Geometry check sheet. Reference: drawing and pictorial views, mm from the part's lowest x, y, z. A direction names the side the tool comes from. Give positions to 0.01 mm unless a question says otherwise; leave off trailing zeros. Write each loop counter-clockwise with the first axis right and the second up, starting at its lowest first coordinate (ties: lowest second). Pieces come first, ordered by that corner, then holes. Notation, with made-up numbers: (9, 77.25) -> (14, 77.25) arc R32 cw to (14, 105.25) -> close; hole circle Ø5 at (82, -38). An arc over 180 degrees is marked (long way). Return JSON: item names as keys, results as strings.
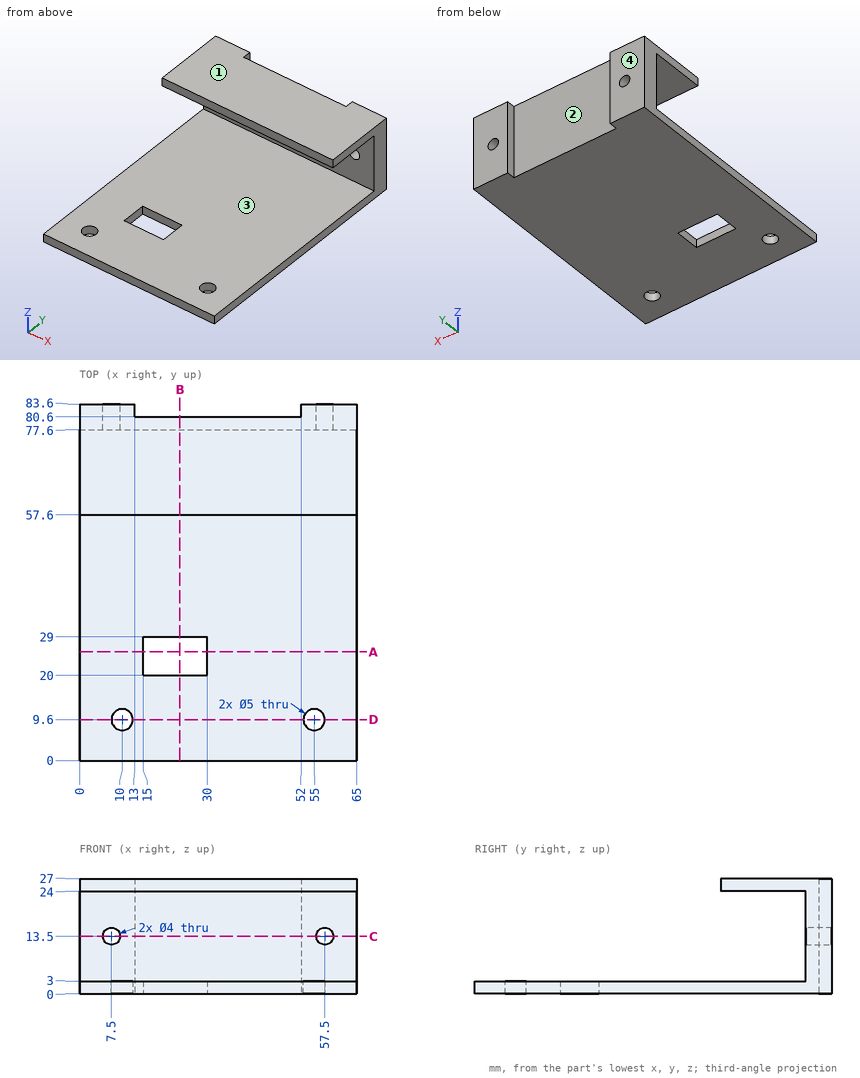
(1) Cross-section at C-C on z = 13.5. Enter the section's corners in (x, y).
Reply:
{"outline": "(0, 77.6) -> (5.5, 77.6) -> (5.5, 83.6) -> (0, 83.6) -> close; (9.5, 77.6) -> (55.5, 77.6) -> (55.5, 83.6) -> (52, 83.6) -> (52, 80.6) -> (13, 80.6) -> (13, 83.6) -> (9.5, 83.6) -> close; (59.5, 77.6) -> (65, 77.6) -> (65, 83.6) -> (59.5, 83.6) -> close"}
(2) Set-up check for the marked faces 3 and 4: record each of +Z, -Z, +X, -X, +Y, -Y from which the full face is reachable in a straight line by a thin tool's end or side.
Reply:
{"face 3": "+X, -X, -Y", "face 4": "+Z, -Z, +X, -X, +Y"}
(3) Release check for a two-part mould opening along X. For the marked faces 1 and 2 record: pulls with the +X half, pulls with the -X half, needs draft (parallel to the pull), parting line crosses it, or undercut.
Reply:
{"face 1": "needs draft", "face 2": "undercut"}
(4) Cross-section at D-D on y = 9.6. Enter the section's corners in (x, z).
Reply:
{"outline": "(0, 0) -> (7.5, 0) -> (7.5, 3) -> (0, 3) -> close; (12.5, 0) -> (52.5, 0) -> (52.5, 3) -> (12.5, 3) -> close; (57.5, 0) -> (65, 0) -> (65, 3) -> (57.5, 3) -> close"}
(5) Cross-section at A-A on y = 25.5. Enter the section's corners in (x, z).
Reply:
{"outline": "(0, 0) -> (15, 0) -> (15, 3) -> (0, 3) -> close; (30, 0) -> (65, 0) -> (65, 3) -> (30, 3) -> close"}
(6) Cross-section at B-B on x = 23.5. Enter the section's corners in (y, z).
Reply:
{"outline": "(0, 0) -> (20, 0) -> (20, 3) -> (0, 3) -> close; (29, 0) -> (80.6, 0) -> (80.6, 27) -> (57.6, 27) -> (57.6, 24) -> (77.6, 24) -> (77.6, 3) -> (29, 3) -> close"}
(7) Thickness scan on L1, parallel to Y at x = 10, z = 1.05; L2, parallel to X at y = 81.9, z = 13.5; L3, parallel to Z at x = 35, y = 58. Record the ranges inside material, lowest first.
Reply:
{"L1": "0 to 7.1, 12.1 to 83.6", "L2": "0 to 5.5, 9.5 to 13, 52 to 55.5, 59.5 to 65", "L3": "0 to 3, 24 to 27"}
(8) Depth check by flat-ended pin: pin 1 Ø0.9 at (x, z) = (47.5, 25) entering from -Y; pin 2 Ø4 at (x, z) = (40, 12) entering from -Y; pin 3 Ø6 at (x, y) = (10, 9.6) entering from +Z. Enter the tip coordinate at first touch or a pass-through.
Reply:
{"pin 1": "y = 57.6", "pin 2": "y = 77.6", "pin 3": "z = 3"}
